Model file for the job. Use its own axes, mm. A direction names the side the tool comes from. Round coordinates to 2 decimals unless told otherwise and drop trailing zeros. Loops run counter-clockwise (first coordinate to the right, second up) from the corner with the lowest first, then second, coordinate; pieces in that order, holes last. Notation, with made-up numbers: (-13.75, -11) -> (19.25, -11) arc R24 cw to (19.25, 28) -> close; hole circle Ø2 at (89, 65.5). An arc over 180 degrees is marked (long way). Use a Markdown table: item, result.
from build123d import *

# Parameters (mm, degrees)
F1_DEPTH  = 12.7
F2_R      = 6.35
F3_T      = -2.54
F4_R      = 3.175
F5_DEPTH  = 2.54
F7_R      = 3.175
F8_DEPTH  = 10.16
F9_R      = 1.5875
F10_DEPTH = 6.35
F11_R     = 22.225
F12_DEPTH = 2.54


with BuildPart() as f1:
    # F0 (on Top) → F1 (new body)
    with BuildSketch(Plane.XY):
        with BuildLine():
            Line((-31.75, -31.75), (31.75, -31.75))
            ThreePointArc((31.75, -31.75), (36.2401280605, -29.8901280605), (38.1, -25.4))
            Line((38.1, -25.4), (38.1, 25.4))
            ThreePointArc((38.1, 25.4), (36.2401280605, 29.8901280605), (31.75, 31.75))
            Line((31.75, 31.75), (-31.75, 31.75))
            ThreePointArc((-31.75, 31.75), (-36.2401280605, 29.8901280605), (-38.1, 25.4))
            Line((-38.1, 25.4), (-38.1, -25.4))
            ThreePointArc((-38.1, -25.4), (-36.2401280605, -29.8901280605), (-31.75, -31.75))
        make_face()
    extrude(amount=F1_DEPTH)

    # F2
    f2_edges = [f1.edges().sort_by_distance(p)[0] for p in [
        (0, -31.75, 12.7),
        (36.240128, -29.890128, 12.7),
        (38.1, 0, 12.7),
        (36.240128, 29.890128, 12.7),
        (0, 31.75, 12.7),
        (-36.240128, 29.890128, 12.7),
        (-38.1, 0, 12.7),
        (-36.240128, -29.890128, 12.7),
    ]]
    fillet(f2_edges, radius=F2_R)

    # F3
    f3_openings = [f1.faces().sort_by_distance(p)[0] for p in [
        (0, 0, 0),
    ]]
    offset(amount=F3_T, openings=f3_openings)

    # F4 (on face) → F5 (cut, through all)
    with BuildSketch(Plane(origin=(-38.1, 0, 0), x_dir=(0, -1, 0), z_dir=(-1, 0, 0))):
        with Locations((19.05, 0)):
            Circle(F4_R)
    extrude(amount=-F5_DEPTH, mode=Mode.SUBTRACT)

    # F7 (on offset) → F8 (join, through all)
    with BuildSketch(Plane(origin=(0, 0, 10.16), x_dir=(1, 0, 0), z_dir=(0, 0, -1))):
        with Locations((-31.5977446735, 25.4)):
            Circle(F7_R)
        with Locations((-31.5977446735, -25.4)):
            Circle(F7_R)
        with Locations((31.9022553265, 25.4)):
            Circle(F7_R)
        with Locations((31.9022553265, -25.4)):
            Circle(F7_R)
    extrude(amount=F8_DEPTH)

    # F9 (on face) → F10 (join)
    with BuildSketch(Plane(origin=(0, 0, 0), x_dir=(1, 0, 0), z_dir=(0, 0, -1))):
        with Locations((-31.5977446735, 25.4)):
            Circle(F9_R)
        with Locations((-31.5977446735, -25.4)):
            Circle(F9_R)
        with Locations((31.9022553265, 25.4)):
            Circle(F9_R)
        with Locations((31.9022553265, -25.4)):
            Circle(F9_R)
    extrude(amount=F10_DEPTH)

    # F11 (on face) → F12 (cut, through all)
    with BuildSketch(Plane.XY.offset(12.7)):
        Circle(F11_R)
    extrude(amount=-F12_DEPTH, mode=Mode.SUBTRACT)


solid = f1.part
Q1. Flat gauge pins, fed straight in: pin 1 (6 mm diameter, centred on y = -2, z = 10, fed in from -X); pin 2 (4 mm diameter, centred on x = -27, y = -22.5, fed in from -Z). Where does each tip first touch, or does it go through?
Results list:
| item | result |
|---|---|
| pin 1 | stops at x = -38.07 |
| pin 2 | stops at z = 10.16 |
Q2. Band-saw the part on C-C, the plane z = 11.25. Give the cut face in (x, y) (3 decimals).
Results list:
| item | result |
|---|---|
| outline | (-35.789, -25.4) arc R4.039 ccw to (-31.75, -29.439) -> (31.75, -29.439) arc R4.039 ccw to (35.789, -25.4) -> (35.789, 25.4) arc R4.039 ccw to (31.75, 29.439) -> (-31.75, 29.439) arc R4.039 ccw to (-35.789, 25.4) -> close; hole circle Ø44.45 at (0, 0) |
Q3. Tool access for faces 4 (the face through (-22, 6, 12.7)), 5 (the face through (-36.848, -19.12, 3.174)), 6 (the face through (-32.77, 24.33, -3.13)): list every direction of +Z, -Z, +X, -X, +Y, -Y with a clear straight run to the whole face (end or side of a thin tool).
Results list:
| item | result |
|---|---|
| face 4 | +Z, +X, -X, +Y, -Y |
| face 5 | -Z, -X |
| face 6 | -Z |
Q4. Drill centre lines: L1, parallel to Y at x = 5, z = 6; L2, parallel to Y at x = 0, z = 11.45 (3 decimals); L3, parallel to Z at x = 29.5, y = 16.5. Where is each one in solid material? Low to high. Write a range as from..to.
Results list:
| item | result |
|---|---|
| L1 | y = -31.75..-29.21, 29.21..31.75 |
| L2 | y = -29.183..-22.225, 22.225..29.183 |
| L3 | z = 10.16..12.7 |
Q5. Band-saw the part on A-A, the plane y = 0. Give the cut face in (x, z) (3 decimals).
Results list:
| item | result |
|---|---|
| outline | (-38.1, 0) -> (-35.56, 0) -> (-35.56, 6.35) arc R3.81 cw to (-31.75, 10.16) -> (-22.225, 10.16) -> (-22.225, 12.7) -> (-31.75, 12.7) arc R6.35 ccw to (-38.1, 6.35) -> close; (22.225, 10.16) -> (31.75, 10.16) arc R3.81 cw to (35.56, 6.35) -> (35.56, 0) -> (38.1, 0) -> (38.1, 6.35) arc R6.35 ccw to (31.75, 12.7) -> (22.225, 12.7) -> close |
Q6. Band-saw the part on D-D, the plane z = -3. Give the cut face in (x, y) (1 decimal), plus the area to 3 significant figures.
Results list:
| item | result |
|---|---|
| outline | circle Ø3.2 at (-31.6, -25.4); circle Ø3.2 at (-31.6, 25.4); circle Ø3.2 at (31.9, -25.4); circle Ø3.2 at (31.9, 25.4) |
| area | 31.7 mm² |
Q7. Pull direction X, two halves, no side cores. Call faces 1 (the face through (30.73, 24.33, -3.13)), 2 (the face through (36.19, -29.94, 3.13)), 3 (the face through (-32, 25, -6.35)): released by +X, released by -X, zero draft, split by the parting line, or undercut.
Results list:
| item | result |
|---|---|
| face 1 | undercut |
| face 2 | released by +X |
| face 3 | zero draft |
Q8. Band-saw the part on B-B, the plane x = 0. Give the cut face in (y, z) (3 decimals).
Results list:
| item | result |
|---|---|
| outline | (-31.75, 0) -> (-29.21, 0) -> (-29.21, 6.35) arc R3.81 cw to (-25.4, 10.16) -> (-22.225, 10.16) -> (-22.225, 12.7) -> (-25.4, 12.7) arc R6.35 ccw to (-31.75, 6.35) -> close; (22.225, 10.16) -> (25.4, 10.16) arc R3.81 cw to (29.21, 6.35) -> (29.21, 0) -> (31.75, 0) -> (31.75, 6.35) arc R6.35 ccw to (25.4, 12.7) -> (22.225, 12.7) -> close |
